Verification items for the finished model (mm, model axes). Give positions to 0.01 mm unless a question says otherwise; leave off trailing zeros. Order: outer loops, then holes, each group sorted by start corner. A loop starts at its lowest first (then second) coordinate and runs counter-clockwise, first axis right, second up. Notation, with made-up numbers: (27.25, 36.25) -> (66.25, 36.25) arc R18 ccw to (66.25, 52.25) -> close; hole circle Ø9 at (-29, 6). An arc over 180 degrees is marked (long way). Return JSON: item names as keys, results as strings. Group by question number.
(1) Cross-section at A-A on z = 0.4. State how many separate pieces and enclosed holes the cut face has, then the cut area to 3 significant figures.
(2) Thickness scan on line 1 along X through (y, z) = (154.5, 1.45); line 2 along Y through (x, z) = (246.5, 0.45); line 3 along X through (y, z) = (62.5, 1.8). Record the ranges inside material, lowest first.
(3) Cross-section at B-B on y = 32.5. Enter the section's corners in (x, z), then the cut area to 3 significant figures.
(4) Depth check by flat-ended pin: pin 1 Ø1 at (y, z) = (98.5, 1) entering from +X; pin 2 Ø0.6 at (x, z) = (269, 0.5) entering from +Y; pin 3 Ø2.5 at (x, y) = (267.75, 154.5) entering from -Z; pin 4 Ø0.6 at (y, z) = (168, 0.5) entering from -X. Enter the tip coordinate at first touch or a pass-through.
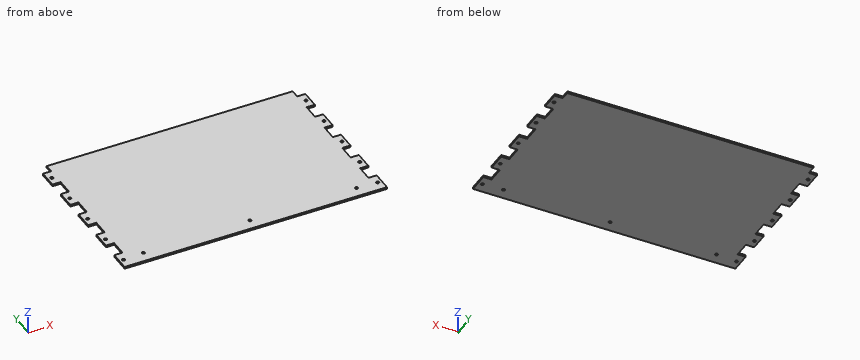
from build123d import *

# Parameters (mm, degrees)
SKETCH1_R           = 1.5
BOSS_EXTRUDE1_DEPTH = 2


with BuildPart() as part:
    # Sketch1 → Boss-Extrude1 (new body)
    with BuildSketch(Plane.XY):
        Polygon((0, 20.8), (8.5, 20.8), (8.5, 37.6), (0, 37.6), (0, 56.6), (8.5, 56.6), (8.5, 73.4), (0, 73.4), (0, 92.4), (8.5, 92.4), (8.5, 109.2), (0, 109.2), (0, 128.2), (8.5, 128.2), (8.5, 145), (0, 145), (0, 164), (8.5, 164), (8.5, 173), (263.5, 173), (263.5, 164), (272, 164), (272, 145), (263.5, 145), (263.5, 128.2), (272, 128.2), (272, 109.2), (263.5, 109.2), (263.5, 92.4), (272, 92.4), (272, 73.4), (263.5, 73.4), (263.5, 56.6), (272, 56.6), (272, 37.6), (263.5, 37.6), (263.5, 20.8), (272, 20.8), (272, 0), (0, 0), align=None)
        with Locations((4.25, 154.5)):
            Circle(SKETCH1_R, mode=Mode.SUBTRACT)
        with Locations((4.25, 118.5)):
            Circle(SKETCH1_R, mode=Mode.SUBTRACT)
        with Locations((4.25, 82.5)):
            Circle(SKETCH1_R, mode=Mode.SUBTRACT)
        with Locations((4.25, 46.5)):
            Circle(SKETCH1_R, mode=Mode.SUBTRACT)
        with Locations((4.25, 10.5)):
            Circle(SKETCH1_R, mode=Mode.SUBTRACT)
        with Locations(Location((267.75, 10.5, 0), (0, 0, 180))):
            Circle(SKETCH1_R, mode=Mode.SUBTRACT)
        with Locations(Location((267.75, 46.5, 0), (0, 0, 180))):
            Circle(SKETCH1_R, mode=Mode.SUBTRACT)
        with Locations(Location((267.75, 82.5, 0), (0, 0, 180))):
            Circle(SKETCH1_R, mode=Mode.SUBTRACT)
        with Locations(Location((267.75, 118.5, 0), (0, 0, 180))):
            Circle(SKETCH1_R, mode=Mode.SUBTRACT)
        with Locations(Location((267.75, 154.5, 0), (0, 0, 180))):
            Circle(SKETCH1_R, mode=Mode.SUBTRACT)
        with Locations((25.5, 11.75)):
            Circle(SKETCH1_R, mode=Mode.SUBTRACT)
        with Locations((136, 11.75)):
            Circle(SKETCH1_R, mode=Mode.SUBTRACT)
        with Locations((246.5, 11.75)):
            Circle(SKETCH1_R, mode=Mode.SUBTRACT)
    extrude(amount=BOSS_EXTRUDE1_DEPTH)


solid = part.part
Verdict:
{
 "1": {"separate pieces": "1", "enclosed holes": "13", "area": "45,700 mm²"},
 "2": {"line 1": "0 to 2.75, 5.75 to 266.25, 269.25 to 272", "line 2": "0 to 10.25, 13.25 to 173", "line 3": "8.5 to 263.5"},
 "3": {"outline": "(8.5, 0) -> (263.5, 0) -> (263.5, 2) -> (8.5, 2) -> close", "area": "510 mm²"},
 "4": {"pin 1": "x = 263.5", "pin 2": "y = 164", "pin 3": "through", "pin 4": "x = 8.5"}
}
